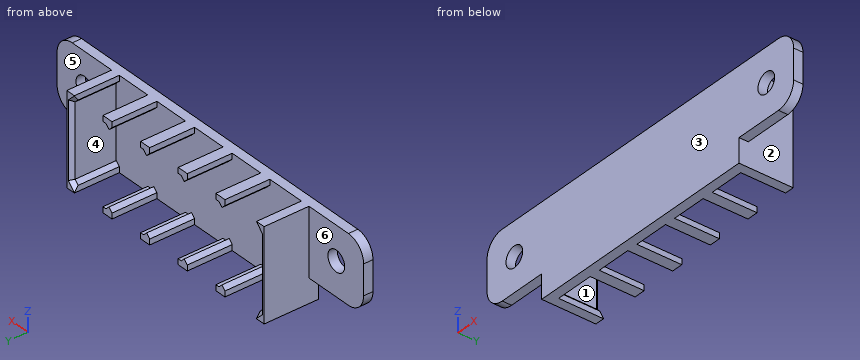
from build123d import *

# Parameters (mm, degrees)
SKETCH_1_W                    = 65
SKETCH_1_H                    = 24.4
EXTRUDE_1_DEPTH               = 2.5
SKETCH_2_R                    = 2.75
EXTRUDE_2_DEPTH               = 2.5
EXTRUDE_3_DEPTH               = 12
CHAMFER_1_SIZE                = 1
EXTRUDE_4_DEPTH               = 12
PATTERN_LINEAR_1_COUNT        = 4
PATTERN_LINEAR_1_PITCH        = 12.4
PATTERN_LINEAR_1_COPY_1_DEPTH = 12
PATTERN_LINEAR_1_COPY_2_DEPTH = 12
PATTERN_LINEAR_1_COPY_3_DEPTH = 12


with BuildPart() as part:
    # Эскиз1 → Бобышка-Вытянуть1 (new body)
    with BuildSketch(Plane(origin=(0, 0, 0), x_dir=(1, 0, 0), z_dir=(0, 1, 0))):
        with Locations((0, 2.228571429)):
            Rectangle(SKETCH_1_W, SKETCH_1_H)
    extrude(amount=EXTRUDE_1_DEPTH)

    # Эскиз2 → Бобышка-Вытянуть2 (add)
    with BuildSketch(Plane(origin=(0, 0, 0), x_dir=(1, 0, 0), z_dir=(0, 1, 0))):
        with BuildLine():
            Line((-32.5, -9.971428571), (-45.5, -9.971428571))
            ThreePointArc((-45.5, -9.971428571), (-49.035533906, -8.506962477), (-50.5, -4.971428571))
            Line((-50.5, -4.971428571), (-50.5, 3.028571429))
            ThreePointArc((-50.5, 3.028571429), (-49.035533906, 6.564105335), (-45.5, 8.028571429))
            Line((-45.5, 8.028571429), (-32.5, 8.028571429))
            Line((-32.5, 8.028571429), (-32.5, -9.971428571))
        make_face()
        with Locations(Location((-41.5, -0.971428571, 0), (0, 0, 270))):
            Circle(SKETCH_2_R, mode=Mode.SUBTRACT)
    extrude_2 = extrude(amount=EXTRUDE_2_DEPTH)

    # Зеркальное отражение1: Бобышка-Вытянуть2 across plane
    add(extrude_2.mirror(Plane(origin=(0, 0, 0), x_dir=(0, 0, 1), z_dir=(1, 0, 0))))

    # Эскиз3 → Бобышка-Вытянуть3 (add)
    with BuildSketch(Plane(origin=(0, 2.5, 0), x_dir=(1, 0, 0), z_dir=(0, 1, 0))):
        Polygon((-32.5, 14.428571429), (-31, 14.428571429), (-30, 14.428571429), (-30, 12.928571429), (-31, 11.928571429), (-31, -7.471428571), (-30, -8.471428571), (-30, -9.971428571), (-31, -9.971428571), (-32.5, -9.971428571), align=None)
    extrude_3 = extrude(amount=EXTRUDE_3_DEPTH)

    # Зеркальное отражение2: Бобышка-Вытянуть3 across plane
    add(extrude_3.mirror(Plane(origin=(0, 0, 0), x_dir=(0, 0, 1), z_dir=(1, 0, 0))))

    # Фаска1
    chamfer_1_edges = [part.edges().sort_by_distance(p)[0] for p in [
        (-30.5, 14.5, 7.971428571),
        (-31, 14.5, -2.228571429),
        (-30.5, 14.5, -12.428571429),
        (30.5, 14.5, -12.428571429),
        (31, 14.5, -2.228571429),
        (30.5, 14.5, 7.971428571),
    ]]
    chamfer(chamfer_1_edges, length=CHAMFER_1_SIZE)

    # Эскиз4 → Бобышка-Вытянуть4 (add)
    with BuildSketch(Plane(origin=(0, 2.5, 0), x_dir=(1, 0, 0), z_dir=(0, 1, 0))):
        Polygon((-18.6, -9.971428571), (-19.6, -9.971428571), (-19.6, -8.471428571), (-18.6, -7.471428571), (-17.6, -8.471428571), (-16.6, -8.471428571), (-16.6, -9.971428571), align=None)
    extrude_4 = extrude(amount=EXTRUDE_4_DEPTH)

    # Зеркальное отражение3: Бобышка-Вытянуть4 across plane
    add(extrude_4.mirror(Plane.XY.offset(-2.228571429)))

    # Линейный массив1: Бобышка-Вытянуть4 ×4
    with Locations(*[(i * PATTERN_LINEAR_1_PITCH, 0, 0) for i in range(1, PATTERN_LINEAR_1_COUNT)]):
        add(extrude_4)

    # Линейный массив1 copy 1 sketch → Линейный массив1 copy 1 (add)
    with BuildSketch(Plane(origin=(12.4, 2.5, -4.457142857), x_dir=(1, 0, 0), z_dir=(0, 1, 0))):
        Polygon((-18.6, 9.971428571), (-19.6, 9.971428571), (-19.6, 8.471428571), (-18.6, 7.471428571), (-17.6, 8.471428571), (-16.6, 8.471428571), (-16.6, 9.971428571), align=None)
    extrude(amount=PATTERN_LINEAR_1_COPY_1_DEPTH)

    # Линейный массив1 copy 2 sketch → Линейный массив1 copy 2 (add)
    with BuildSketch(Plane(origin=(24.8, 2.5, -4.457142857), x_dir=(1, 0, 0), z_dir=(0, 1, 0))):
        Polygon((-18.6, 9.971428571), (-19.6, 9.971428571), (-19.6, 8.471428571), (-18.6, 7.471428571), (-17.6, 8.471428571), (-16.6, 8.471428571), (-16.6, 9.971428571), align=None)
    extrude(amount=PATTERN_LINEAR_1_COPY_2_DEPTH)

    # Линейный массив1 copy 3 sketch → Линейный массив1 copy 3 (add)
    with BuildSketch(Plane(origin=(37.2, 2.5, -4.457142857), x_dir=(1, 0, 0), z_dir=(0, 1, 0))):
        Polygon((-18.6, 9.971428571), (-19.6, 9.971428571), (-19.6, 8.471428571), (-18.6, 7.471428571), (-17.6, 8.471428571), (-16.6, 8.471428571), (-16.6, 9.971428571), align=None)
    extrude(amount=PATTERN_LINEAR_1_COPY_3_DEPTH)


solid = part.part
Check sheet for the modelled part. Datum: model origin and axes. Units: mm. Face numbers are marked on the shaded views. A direction names the side the tool comes from. Round coordinates to 2 decimals unless told otherwise and drop trailing zeros. Order: outer loops, then holes, each group sorted by start corner. A loop starts at its lowest first (then second) coordinate and runs counter-clockwise, first axis right, second up. Notation, with made-up numbers: M 58.25,65 L 109.25,65 A8 cw 109.25,78 Z; hole C 75,83.25 d8. An arc over 180 degrees is marked long. One line per item, written item: value. Start each with the question number.
1. Gauge pin test, flat ends, axial feed: P1, Ø1.6, axis at y = 6, z = 9.5, coming from the +X side; P2, Ø1, axis at x = -4.5, z = -6.5, coming from the +Y side; P3, Ø3, axis at x = 36, y = 1.5, coming from the -Z side. Record the tip position at first contact, or that the pin passes through.
2. Section check C-C on y = 1.5. Enter the section's corners in (x, z).
3. Section check D-D on x = 15. Enter the section's corners in (y, z), and give its area (3 significant figures).
4. Section check A-A on x = -41.5. Enter the section's corners in (y, z).
5. Scan lines: line 1 along X through (y, z) = (4.5, 0.25); line 2 along Y through (x, z) = (-14.5, -6.75); line 3 along Z through (x, y) = (5.5, 7.25). Record each from-to range of solid material in increasing order.
6. Access from +Z, -Z, +X, -X, +Y, -Y to the whole of each face (thin tool, end or side, straight path). Record for the marked faces 3, 4, 5 and 6.
7. Section check B-B on z = 2.75. Enter the section's corners in (x, y), and give its area (3 significant figures).
8. Release check for a two-part mould opening along Z. For the marked faces 1 and 2 record: released by +Z, released by -Z, zero draft, split by the parting line, or undercut.
Results found:
1. P1: x = 32.5
1. P2: y = 2.5
1. P3: z = -8.03
2. outline: M -50.5,-3.03 A5 ccw -45.5,-8.03 L -32.5,-8.03 L -32.5,-14.43 L 32.5,-14.43 L 32.5,-8.03 L 45.5,-8.03 A5 ccw 50.5,-3.03 L 50.5,4.97 A5 ccw 45.5,9.97 L -45.5,9.97 A5 ccw -50.5,4.97 Z; hole C -41.5,0.97 d5.5; hole C 41.5,0.97 d5.5
3. outline: M 0,-14.43 L 2.5,-14.43 L 2.5,9.97 L 0,9.97 Z
3. area: 61.0 mm^2
4. outline: M 0,-8.03 L 2.5,-8.03 L 2.5,-1.78 L 0,-1.78 Z; M 0,3.72 L 2.5,3.72 L 2.5,9.97 L 0,9.97 Z
5. line 1: -32.5 to -31, 31 to 32.5
5. line 2: 0 to 2.5
5. line 3: -14.43 to -12.63, 8.17 to 9.97
6. face 3: +Z, -Z, +X, -X, -Y
6. face 4: +Y
6. face 5: +Z, -Z, +X, +Y
6. face 6: +Z, -Z, -X, +Y
7. outline: M -50.5,0 L -43.6,0 L -43.6,2.5 L -50.5,2.5 Z; M -39.4,0 L 39.4,0 L 39.4,2.5 L 32.5,2.5 L 32.5,14.5 L 32,14.5 L 31,13.5 L 31,2.5 L -31,2.5 L -31,13.5 L -32,14.5 L -32.5,14.5 L -32.5,2.5 L -39.4,2.5 Z; M 43.6,0 L 50.5,0 L 50.5,2.5 L 43.6,2.5 Z
7. area: 267 mm^2
8. face 1: undercut
8. face 2: zero draft
